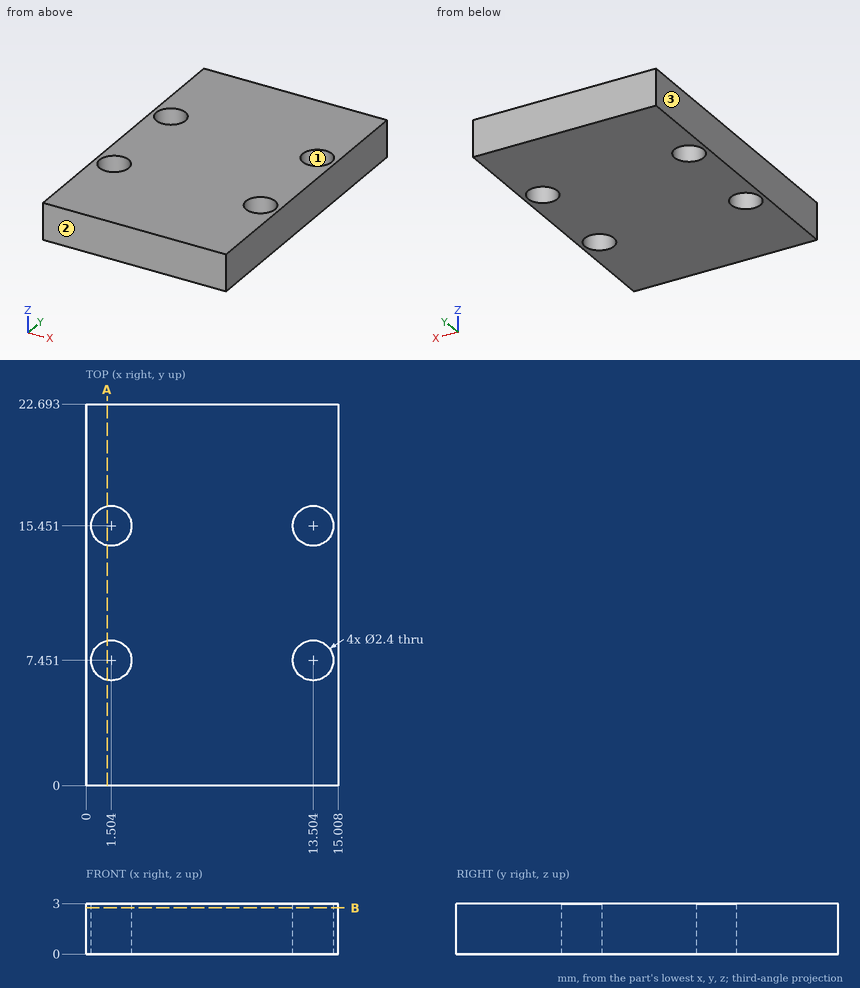
Source: three-view drawing plus pictorial views. Frame: mm from the lowest corner of the part. Give positions to 0.01 mm unless a question says otherwise; leave off trailing zeros. Order: outer loops, then holes, each group sorted by start corner. A loop starts at its lowest first (then second) coordinate and runs counter-clockwise, first axis right, second up. Notation, with made-up numbers: M 18,-3.75 L 68,-3.75 A18 cw 68,13.25 Z; hole C -14.75,-32.5 d1. An arc over 180 degrees is marked long. Return JSON: item names as keys, results as strings.
1) Line query: L1, parallel to Y at x = 1.5, z = 2.4; L2, parallel to X at y = 15.25, z = 2.5; L3, parallel to Y at x = 14, z = 2.6 (1 decimal). Output: solid intervals per line, ascending. Write a range as [from, to].
Taken from the geometry:
{"L1": "y = [0, 6.25], [8.65, 14.25], [16.65, 22.69]", "L2": "x = [0, 0.32], [2.69, 12.32], [14.69, 15.01]", "L3": "y = [0, 6.4], [8.5, 14.4], [16.5, 22.7]"}
2) Section query A-A on x = 1.25. Output: boundary loops of the cut face in (y, z).
Taken from the geometry:
{"outline": "M 0,0 L 6.28,0 L 6.28,3 L 0,3 Z; M 8.62,0 L 14.28,0 L 14.28,3 L 8.62,3 Z; M 16.62,0 L 22.69,0 L 22.69,3 L 16.62,3 Z"}
3) Mould query, pull axis X, two halves, no side actions, for the marked faces 1, 2 and 3. Classes: released by +X, released by -X, zero draft, split by the parting line, or undercut.
Taken from the geometry:
{"face 1": "undercut", "face 2": "zero draft", "face 3": "released by -X"}
4) Section query B-B on z = 2.75. Count the separate pieces of the cut face and the enclosed holes in it.
Taken from the geometry:
{"separate pieces": "1", "enclosed holes": "4"}
